Check sheet for the drawn part. Datum: minimum x, y, z corner. Units: mm. Round coordinates to 2 decimals unless told otherwise and drop trailing zeros. Write each loop counter-clockwise with the first axis right and the second up, starting at its lowest first coordinate (ties: lowest second). Pieces come first, ordered by that corner, then holes. Notation, with made-up numbers: (88.5, -23) -> (139.5, -23) arc R16 cw to (139.5, -4) -> close; hole circle Ø9 at (46.5, -11). An arc over 180 degrees is marked (long way). Use a Markdown table: item, result.
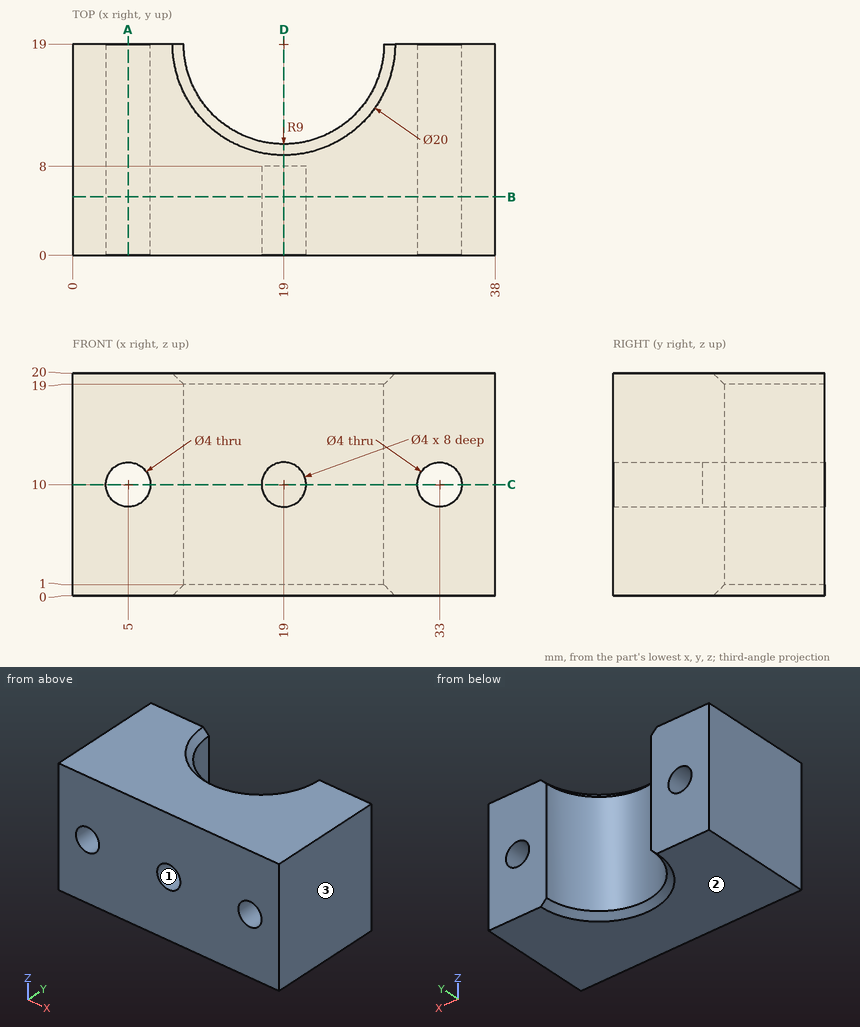
(1) Section check C-C on z = 10. Record the cut outline in (x, y), plus the area to 3 significant figures.
A:
| item | result |
|---|---|
| outline | (0, 0) -> (3, 0) -> (3, 19) -> (0, 19) -> close; (7, 0) -> (17, 0) -> (17, 8) -> (21, 8) -> (21, 0) -> (31, 0) -> (31, 19) -> (28, 19) arc R9 cw to (10, 19) -> (7, 19) -> close; (35, 0) -> (38, 0) -> (38, 19) -> (35, 19) -> close |
| area | 411 mm2 |
(2) Gauge pin test, flat ends, axial feed: pin 1 Ø6.5 at (x, z) = (19, 10) entering from +Y; pin 2 Ø6.5 at (x, z) = (5, 10) entering from -Y; pin 3 Ø1 at (x, z) = (16.5, 9) entering from +Y. Record the tip position at first contact, or that the pin passes through.
A:
| item | result |
|---|---|
| pin 1 | stops at y = 10.61 |
| pin 2 | stops at y = 0 |
| pin 3 | stops at y = 10.51 |
(3) Section check A-A on x = 5. Record the cut outline in (y, z), plus the area to 3 significant figures.
A:
| item | result |
|---|---|
| outline | (0, 0) -> (19, 0) -> (19, 8) -> (0, 8) -> close; (0, 12) -> (19, 12) -> (19, 20) -> (0, 20) -> close |
| area | 304 mm2 |
(4) Release check for a two-part mould opening along Z. For the marked faces 1, 2 and 3 record: +Z half, -Z half, draft (parallel to the pull), parting line (faces both ways), or undercut.
A:
| item | result |
|---|---|
| face 1 | undercut |
| face 2 | -Z half |
| face 3 | draft |
(5) Section check D-D on x = 19. Record the cut outline in (y, z), plus the area to 3 significant figures.
A:
| item | result |
|---|---|
| outline | (0, 0) -> (9, 0) -> (10, 1) -> (10, 19) -> (9, 20) -> (0, 20) -> (0, 12) -> (8, 12) -> (8, 8) -> (0, 8) -> close |
| area | 167 mm2 |
(6) Thickness scan on line 1 (Z direction, x = 33, y = 12.25); line 2 (X direction, y = 6, z = 9.5); line 3 (Z direction, x = 33.5, y = 14.75). Record the ranges inside material, lowest first.
A:
| item | result |
|---|---|
| line 1 | z = 0 to 8, 12 to 20 |
| line 2 | x = 0 to 3.06, 6.94 to 17.06, 20.94 to 31.06, 34.94 to 38 |
| line 3 | z = 0 to 8.06, 11.94 to 20 |
(7) Section check B-B on y = 5.25. Record the cut outline in (x, z), plus the area to 3 significant figures.
A:
| item | result |
|---|---|
| outline | (0, 0) -> (38, 0) -> (38, 20) -> (0, 20) -> close; hole circle Ø4 at (5, 10); hole circle Ø4 at (19, 10); hole circle Ø4 at (33, 10) |
| area | 722 mm2 |
